Build history of the part. All positions in model axes, mm. A direction names the side the tool comes from. Give positions to 0.01 mm unless a question says otherwise; leave off trailing zeros. Order: outer loops, then holes, each group sorted by start corner. A loop starts at its lowest first (then second) coordinate and runs counter-clockwise, first axis right, second up. Notation, with made-up numbers: (-21.5, 36) - (-12.5, 36) arc R10 cw to (-12.5, 46) - close; hole circle Ø8 at (50, 18). An arc over 180 degrees is marked (long way). Answer in a Markdown table with one row per item.
Autodesk Inventor part; units mm, degrees
ref_plane "YZ Plane" through (0, 0, 0) normal (1, 0, 0) x (0, 1, 0)
ref_plane "XZ Plane" through (0, 0, 0) normal (0, 1, 0) x (-1, 0, 0)
ref_plane "XY Plane" through (0, 0, 0) normal (0, 0, 1) x (1, 0, 0)
sketch "Sketch1" plane through (0, 0, 0) normal (0, 0, 1) x (1, 0, 0)
  line L0 (0, 0) -> (-47.5, 0)
  line L1 (-47.5, 0) -> (-72.2487, -24.7487)
  line L2 (-100.4666, 3.6019) -> (-75, 29.0685)
  line L3 (-75, 29.0685) -> (-75, 76.5685)
  line L4 (0, -71.4752) -> (0, 224.6123)
  arc A0 (-100.4666, 3.6019) -> (-72.2487, -24.7487) centre (-66, 9.6889) ccw
  line L5 (-75, 76.5685) -> (0, 76.5685)
  line L6 (0, 153.1371) -> (-47.5, 153.1371)
  line L7 (-47.5, 153.1371) -> (-72.2487, 177.8858)
  line L8 (-100.4666, 149.5352) -> (-75, 124.0685)
  line L9 (-75, 124.0685) -> (-75, 76.5685)
  arc A1 (-72.2487, 177.8858) -> (-100.4666, 149.5352) centre (-66, 143.4481) ccw
  line L10 (0, 0) -> (47.5, 0)
  line L11 (47.5, 0) -> (72.2487, -24.7487)
  line L12 (100.4666, 3.6019) -> (75, 29.0685)
  line L13 (75, 29.0685) -> (75, 76.5685)
  arc A2 (72.2487, -24.7487) -> (100.4666, 3.6019) centre (66, 9.6889) ccw
  line L14 (75, 124.0685) -> (75, 76.5685)
  line L15 (100.4666, 149.5352) -> (75, 124.0685)
  arc A3 (100.4666, 149.5352) -> (72.2487, 177.8858) centre (66, 143.4481) ccw
  line L16 (47.5, 153.1371) -> (72.2487, 177.8858)
  line L17 (0, 153.1371) -> (47.5, 153.1371)
  line L18 (-100.4666, 3.6019) -> (-72.2487, -24.7487)
  line L19 (-75, 29.0685) -> (-47.5, 0)
  circle A4 centre (-74.6902, 1.0941) radius 9
  circle A5 centre (-74.6902, 152.043) radius 9
  circle A6 centre (74.6902, 1.0941) radius 9
  circle A7 centre (74.6902, 152.043) radius 9
  dimension "d0" = 135
  dimension "d1" = 47.5
  dimension "d2" = 35
  dimension "d3" = 40
  dimension "d4" = 75
  dimension "d5" = 35
  dimension "d6" = 66
  dimension "d11" = 20
  dimension "d12" = 38
  dimension "d13" = 18
extrude "Extrusion1" add sketch "Sketch1" along normal blind 1.5 and the other way blind 1.5 contours L0 L19 L3 L5 L4 | L4 L17 L16 A3 L15 L14 L13 L12 A2 L11 L10 | L1 L18 L2 L19 | L5 L9 L8 A1 L7 L6 L4 | A0 L18 | A4 | A5 | A6 | A7
extrude "Extrusion2" add sketch "Sketch1" along normal mid plane 3.2 contours A4 | A5 | A6 | A7
sketch "Sketch2" plane through (0, 0, 1.5) normal (0, 0, 1) x (1, 0, 0)
  point P0 (0, 0)
sketch "Sketch3" plane through (0, 0, 1.5) normal (0, 0, 1) x (1, 0, 0)
  line L0 (0, 20) -> (-35, 20)
  line L1 (-35, 20) -> (-35, 28)
  line L2 (-35, 28) -> (0, 28)
  line L3 (0, 43) -> (-35, 43)
  line L4 (-35, 43) -> (-35, 51)
  line L5 (-35, 51) -> (0, 51)
  line L6 (0, 0) -> (0, 150)
  line L7 (-75, 124.0685) -> (-75, 29.0685)
  line L8 (-75, 76.5685) -> (75, 76.5685)
  line L9 (75, 124.0685) -> (75, 29.0685)
  line L10 (0, 133.1371) -> (-35, 133.1371)
  line L11 (-35, 133.1371) -> (-35, 125.1371)
  line L12 (-35, 125.1371) -> (0, 125.1371)
  line L13 (0, 110.1371) -> (-35, 110.1371)
  line L14 (-35, 110.1371) -> (-35, 102.1371)
  line L15 (-35, 102.1371) -> (0, 102.1371)
  line L16 (0, 20) -> (35, 20)
  line L17 (35, 20) -> (35, 28)
  line L18 (35, 28) -> (0, 28)
  line L19 (0, 43) -> (35, 43)
  line L20 (35, 43) -> (35, 51)
  line L21 (35, 51) -> (0, 51)
  line L22 (35, 102.1371) -> (0, 102.1371)
  line L23 (0, 110.1371) -> (35, 110.1371)
  line L24 (35, 110.1371) -> (35, 102.1371)
  line L25 (35, 125.1371) -> (0, 125.1371)
  line L26 (35, 133.1371) -> (35, 125.1371)
  line L27 (0, 133.1371) -> (35, 133.1371)
  dimension "d21" = 35
  dimension "d22" = 8
  dimension "d23" = 150
  dimension "d24" = 15
  dimension "d25" = 20
extrude "Extrusion3" cut sketch "Sketch3" against normal blind 10
properties part number "Superior_Base"
1. Two-plate mould, pull along Y, no slides. Class faces 5 (the face through (87.91, 16.16, -0.02)), 6 (the face through (-91.016, 167.927, -0.021)), 7 (the face through (-87.91, 16.16, -0.02)), 8 (the face through (91.016, -14.789, -0.021)): +Y half, -Y half, draft (parallel to the pull), parting line (faces both ways), or undercut.
Check result:
| item | result |
|---|---|
| face 5 | undercut |
| face 6 | +Y half |
| face 7 | undercut |
| face 8 | -Y half |
2. Cut at C-C on y = -3.5. Write the cut outline in (x, z), and give its area (3 significant figures).
Check result:
| item | result |
|---|---|
| outline | (-98.42, -1.5) - (-82.43, -1.5) - (-82.43, -1.6) - (-66.95, -1.6) - (-66.95, -1.5) - (-51, -1.5) - (-51, 1.5) - (-66.95, 1.5) - (-66.95, 1.6) - (-82.43, 1.6) - (-82.43, 1.5) - (-98.42, 1.5) - close; (51, -1.5) - (66.95, -1.5) - (66.95, -1.6) - (82.43, -1.6) - (82.43, -1.5) - (98.42, -1.5) - (98.42, 1.5) - (82.43, 1.5) - (82.43, 1.6) - (66.95, 1.6) - (66.95, 1.5) - (51, 1.5) - close |
| area | 291 mm² |
3. Cut at D-D on y = 92.5. Write the cut outline in (x, z), and give its area (3 significant figures).
Check result:
| item | result |
|---|---|
| outline | (-75, -1.5) - (75, -1.5) - (75, 1.5) - (-75, 1.5) - close |
| area | 450 mm² |
4. Cut at B-B on z = -0.4. Count the separate pieces of the cut face and the enclosed holes in it, and give its area (3 significant figures).
Check result:
| item | result |
|---|---|
| separate pieces | 1 |
| enclosed holes | 4 |
| area | 25,500 mm² |
5. Drop flat-ended pins along their axis: P1, Ø1.5, axis at x = 9, z = 0, coming from the +Y side; P2, Ø8, axis at x = -11, y = 144, coming from the +Z side; P3, Ø1.5, axis at x = -54, z = 0, coming from the -Y side. Give the stop position or say it passes through.
Check result:
| item | result |
|---|---|
| P1 | stops at y = 153.14 |
| P2 | stops at z = 1.5 |
| P3 | stops at y = -7.25 |
6. Cut at A-A on x = -31. Write the cut outline in (y, z).
Check result:
| item | result |
|---|---|
| outline | (0, -1.5) - (20, -1.5) - (20, 1.5) - (0, 1.5) - close; (28, -1.5) - (43, -1.5) - (43, 1.5) - (28, 1.5) - close; (51, -1.5) - (102.14, -1.5) - (102.14, 1.5) - (51, 1.5) - close; (110.14, -1.5) - (125.14, -1.5) - (125.14, 1.5) - (110.14, 1.5) - close; (133.14, -1.5) - (153.14, -1.5) - (153.14, 1.5) - (133.14, 1.5) - close |
7. Which spindle directions (+Z, -Z, +X, -X, +Y, -Y) get a long thin tool onto all of the face, cutting with end or side? Do faces 1 (the face through (-59.7, -12.2, 0)), 2 (the face through (75, 152, -1.6)), 3 (the face through (87.91, 136.98, -0.02)), 4 (the face through (-59.701, 165.338, -0.021)). Say none if no direction does.
Check result:
| item | result |
|---|---|
| face 1 | +Z, -Z, -Y |
| face 2 | -Z, +X, -X, +Y, -Y |
| face 3 | +Z, -Z, +X |
| face 4 | +Z, -Z, +Y |
8. Probe line 1 (Y direction, x = -9, z = -0.9); line 2 (X direction, y = 36, z = 1.1); line 3 (Z direction, x = 15, y = 16). List the from-to ranges inside material, lowest first.
Check result:
| item | result |
|---|---|
| line 1 | y = 0 to 20, 28 to 43, 51 to 102.14, 110.14 to 125.14, 133.14 to 153.14 |
| line 2 | x = -75 to 75 |
| line 3 | z = -1.5 to 1.5 |
